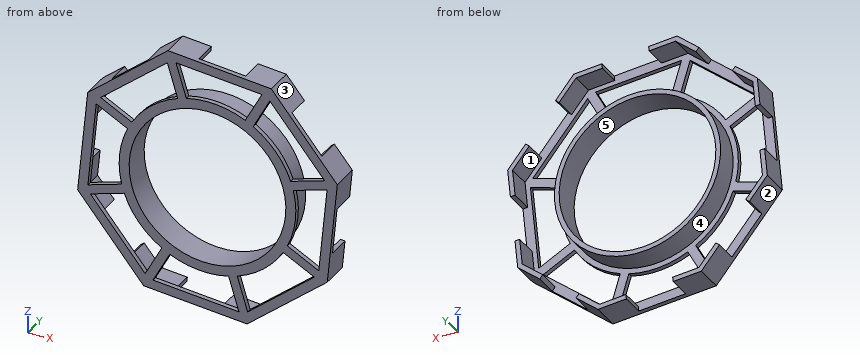
```python
from build123d import *

# Parameters (mm, degrees)
SKETCH1_R           = 50
BOSS_EXTRUDE1_DEPTH = 18
SHELL1_T            = -3
CUT_EXTRUDE1_DEPTH  = 15
CUT_EXTRUDE2_DEPTH  = 119.097158392


with BuildPart() as part:
    # Sketch1 → Boss-Extrude1 (new body)
    with BuildSketch(Plane(origin=(0, 0, 0), x_dir=(1, 0, 0), z_dir=(0, 1, 0))):
        Polygon((-40.722412876, 76.418266738), (-82.830968907, 25.240780326), (-76.418266738, -40.722412876), (-25.240780326, -82.830968907), (40.722412876, -76.418266738), (82.830968907, -25.240780326), (76.418266738, 40.722412876), (25.240780326, 82.830968907), align=None)
        with Locations(Location((0, 0, 0), (0, 0, 270))):
            Circle(SKETCH1_R, mode=Mode.SUBTRACT)
    extrude(amount=BOSS_EXTRUDE1_DEPTH)

    # Shell1
    shell1_openings = [part.faces().sort_by_distance(p)[0] for p in [
        (-59.967550003, 18, -49.340972299),
    ]]
    offset(amount=SHELL1_T, openings=shell1_openings, kind=Kind.INTERSECTION)

    # Sketch3 → Cut-Extrude1 (cut)
    with BuildSketch(Plane(origin=(0, 18, 0), x_dir=(1, 0, 0), z_dir=(0, 1, 0))):
        Polygon((7.118415409, 81.069178382), (7.408696019, 78.083255213), (-22.450535664, 75.18044911), (-22.740816275, 78.166372279), align=None)
        Polygon((60.451938453, 49.974460064), (37.285679369, 69.035531388), (39.191786502, 71.352157297), (62.358045586, 52.291085972), align=None)
        Polygon((78.083255213, -7.408696019), (75.18044911, 22.450535664), (78.166372279, 22.740816275), (81.069178382, -7.118415409), align=None)
        Polygon((49.974460064, -60.451938453), (69.035531388, -37.285679369), (71.352157297, -39.191786502), (52.291085972, -62.358045586), align=None)
        Polygon((-7.408696019, -78.083255213), (22.450535664, -75.18044911), (22.740816275, -78.166372279), (-7.118415409, -81.069178382), align=None)
        Polygon((-60.451938453, -49.974460064), (-37.285679369, -69.035531388), (-39.191786502, -71.352157297), (-62.358045586, -52.291085972), align=None)
        Polygon((-78.083255213, 7.408696019), (-75.18044911, -22.450535664), (-78.166372279, -22.740816275), (-81.069178382, 7.118415409), align=None)
        Polygon((-49.974460064, 60.451938453), (-69.035531388, 37.285679369), (-71.352157297, 39.191786502), (-52.291085972, 62.358045586), align=None)
    extrude(amount=-CUT_EXTRUDE1_DEPTH, mode=Mode.SUBTRACT)

    # Sketch5 → Cut-Extrude2 (cut, through all)
    with BuildSketch(Plane(origin=(0, 3, 0), x_dir=(1, 0, 0), z_dir=(0, 1, 0))):
        with BuildLine():
            Line((-34.746953293, 70.970892834), (-24.087191321, 50.967153462))
            ThreePointArc((-24.087191321, 50.967153462), (-5.614880768, 56.092037151), (13.506743194, 54.730351781))
            Line((13.506743194, 54.730351781), (20.079875719, 76.300958107))
            Line((20.079875719, 76.300958107), (-34.746953293, 70.970892834))
        make_face()
        with BuildLine():
            Line((25.614193291, 74.753805889), (68.151541175, 39.754308602))
            Line((68.151541175, 39.754308602), (48.250912585, 29.149493176))
            ThreePointArc((48.250912585, 29.149493176), (35.692739573, 43.633380106), (19.007003508, 53.071436154))
            Line((19.007003508, 53.071436154), (25.614193291, 74.753805889))
        make_face()
        with BuildLine():
            Line((70.970892834, 34.746953293), (76.300958107, -20.079875719))
            Line((76.300958107, -20.079875719), (54.730351781, -13.506743194))
            ThreePointArc((54.730351781, -13.506743194), (56.092037151, 5.614880768), (50.967153462, 24.087191321))
            Line((50.967153462, 24.087191321), (70.970892834, 34.746953293))
        make_face()
        with BuildLine():
            Line((74.753805889, -25.614193291), (39.754308602, -68.151541175))
            Line((39.754308602, -68.151541175), (29.149493176, -48.250912585))
            ThreePointArc((29.149493176, -48.250912585), (43.633380106, -35.692739573), (53.071436154, -19.007003508))
            Line((53.071436154, -19.007003508), (74.753805889, -25.614193291))
        make_face()
        with BuildLine():
            Line((34.746953293, -70.970892834), (-20.079875719, -76.300958107))
            Line((-20.079875719, -76.300958107), (-13.506743194, -54.730351781))
            ThreePointArc((-13.506743194, -54.730351781), (5.614880768, -56.092037151), (24.087191321, -50.967153462))
            Line((24.087191321, -50.967153462), (34.746953293, -70.970892834))
        make_face()
        with BuildLine():
            Line((-25.614193291, -74.753805889), (-68.151541175, -39.754308602))
            Line((-68.151541175, -39.754308602), (-48.250912585, -29.149493176))
            ThreePointArc((-48.250912585, -29.149493176), (-35.692739573, -43.633380106), (-19.007003508, -53.071436154))
            Line((-19.007003508, -53.071436154), (-25.614193291, -74.753805889))
        make_face()
        with BuildLine():
            Line((-70.970892834, -34.746953293), (-76.300958107, 20.079875719))
            Line((-76.300958107, 20.079875719), (-54.730351781, 13.506743194))
            ThreePointArc((-54.730351781, 13.506743194), (-56.092037151, -5.614880768), (-50.967153462, -24.087191321))
            Line((-50.967153462, -24.087191321), (-70.970892834, -34.746953293))
        make_face()
        with BuildLine():
            Line((-74.753805889, 25.614193291), (-39.754308602, 68.151541175))
            Line((-39.754308602, 68.151541175), (-29.149493176, 48.250912585))
            ThreePointArc((-29.149493176, 48.250912585), (-43.633380106, 35.692739573), (-53.071436154, 19.007003508))
            Line((-53.071436154, 19.007003508), (-74.753805889, 25.614193291))
        make_face()
    extrude(amount=-CUT_EXTRUDE2_DEPTH, mode=Mode.SUBTRACT)


solid = part.part
```
CAD build for the part. Positions are in the model's coordinates, mm. Face numbers are marked on the shaded views. A direction names the side the tool comes from. Round coordinates to 2 decimals unless told otherwise and drop trailing zeros. Order: outer loops, then holes, each group sorted by start corner. A loop starts at its lowest first (then second) coordinate and runs counter-clockwise, first axis right, second up.
Q1. Drop flat-ended pins along their axis: pin 1 (1.5 mm diameter, centred on x = 4, y = 7.5, fed in from +Z); pin 2 (2 mm diameter, centred on y = 14, z = 30.5, fed in from +X); pin 3 (5 mm diameter, centred on x = -22, y = 6, fed in from +Z). Give the stop position or say it passes through.
Q2. Which spindle directions (+Z, -Z, +X, -X, +Y, -Y) get a long thin tool onto all of the face, cutting with end or side? Do the marked faces 4 and 5. Say none if no direction does.
Q3. Slice it at C-C (z = -43.5). Write the cut outline in (x, y), and give its area (3 significant figures).
Q4. Slice it at A-A (y = 11.75). State how many separate pieces and enclosed holes the cut face has, and give its area (3 significant figures).
Q5. Wall check: L1, parallel to X at y = 11, z = 0; L2, parallel to Z at x = -34.5, y = 10; L3, parallel to Z at x = -33, y = 4.5. Give the ranges that are in metal, low to high.
Q6. Slice it at D-D (z = 0). Write the cut outline in (x, y), and give its area (3 significant figures).
Q7. Slice it at B-B (x = 10.5). Write the cut outline in (y, z).
Q8. Two-plate mould, pull along X, no slides. Class the marked faces 1, 2 and 3: pulls with the +X half, pulls with the -X half, needs draft (parallel to the pull), parting line crosses it, or undercut.
Results below:
1. pin 1: stops at z = 52.9
1. pin 2: stops at x = 79.33
1. pin 3: stops at z = 82.76
2. face 4: +Y
2. face 5: +Y, -Y
3. outline: (-67.81, 0) - (-60.04, 0) - (-60.04, 3) - (-67.81, 3) - close; (-35.86, 0) - (-24.65, 0) - (-24.65, 18) - (-30.28, 18) - (-30.28, 3) - (-35.86, 3) - close; (24.65, 0) - (35.86, 0) - (35.86, 3) - (30.28, 3) - (30.28, 18) - (24.65, 18) - close; (63.6, 0) - (73.04, 0) - (73.04, 18) - (68.32, 18) - (68.32, 3) - (63.6, 3) - close
3. area: 358 mm2
4. separate pieces: 9
4. enclosed holes: 1
4. area: 1,810 mm2
5. L1: x = -53 to -50, 50 to 53
5. L2: z = -77.02 to -74.01, -40.23 to -36.19, 36.19 to 40.23, 71.33 to 75.21
5. L3: z = -77.17 to -74.15, -41.47 to -37.56, 37.56 to 41.47, 72.56 to 76.45
6. outline: (-80.38, 0) - (-74.35, 0) - (-74.35, 3) - (-80.38, 3) - close; (-56.37, 0) - (-50, 0) - (-50, 18) - (-53, 18) - (-53, 3) - (-56.37, 3) - close; (50, 0) - (56.37, 0) - (56.37, 3) - (53, 3) - (53, 18) - (50, 18) - close; (74.35, 0) - (80.38, 0) - (80.38, 3) - (74.35, 3) - close
6. area: 164 mm2
7. outline: (0, -81.4) - (18, -81.4) - (18, -78.38) - (3, -78.38) - (3, -75.37) - (0, -75.37) - close; (0, -55.39) - (3, -55.39) - (3, -51.95) - (18, -51.95) - (18, -48.89) - (0, -48.89) - close; (0, 48.89) - (18, 48.89) - (18, 51.95) - (3, 51.95) - (3, 55.39) - (0, 55.39) - close; (0, 73.33) - (3, 73.33) - (3, 79.36) - (0, 79.36) - close
8. face 1: undercut
8. face 2: pulls with the -X half
8. face 3: pulls with the +X half
